```python
from build123d import *

# Parameters (mm, degrees)
SALIENTE_EXTRUIR1_DEPTH = 2
SALIENTE_EXTRUIR2_DEPTH = 24
CROQUIS4_W              = 26.838471133
CROQUIS4_H              = 17.040828642
CORTAR_EXTRUIR1_DEPTH   = 70.1
SALIENTE_EXTRUIR3_DEPTH = 2
SALIENTE_EXTRUIR4_DEPTH = 2
CROQUIS7_W              = 45.5
CROQUIS7_H              = 2
SALIENTE_EXTRUIR5_DEPTH = 8
SALIENTE_EXTRUIR6_DEPTH = 6
CROQUIS9_W              = 76.962380363
CROQUIS9_H              = 58.957858246
CORTAR_EXTRUIR2_DEPTH   = 39


with BuildPart() as part:
    # Croquis1 → Saliente-Extruir1 (new body)
    with BuildSketch(Plane.XY):
        Polygon((-48.939551095, 26.503456625), (-8.439551095, 26.503456625), (-4.439551095, 26.503456625), (-4.439551095, 1.503456625), (-8.439551095, 1.503456625), (-49.939551095, 1.503456625), (-49.939551095, 5.503456625), (-49.939551095, 26.503456625), align=None)
    extrude(amount=SALIENTE_EXTRUIR1_DEPTH)

    # Croquis3 → Saliente-Extruir2 (add)
    with BuildSketch(Plane.XY):
        Polygon((-48.939551095, 26.503456625), (-8.439551095, 26.503456625), (-4.439551095, 26.503456625), (-4.439551095, 1.503456625), (-49.939551095, 1.503456625), (-49.939551095, 26.503456625), align=None)
        Polygon((-10.439551095, 3.503456625), (-47.939551095, 3.503456625), (-47.939551095, 5.503456625), (-47.939551095, 24.503456625), (-10.439551095, 24.503456625), (-6.439551095, 24.503456625), (-6.439551095, 3.503456625), align=None, mode=Mode.SUBTRACT)
    extrude(amount=SALIENTE_EXTRUIR2_DEPTH)

    # Croquis4 → Cortar-Extruir1 (cut)
    with BuildSketch(Plane(origin=(0, 0, 0), x_dir=(0, 0, -1), z_dir=(1, 0, 0))):
        with Locations((-15.419235567, 13.92807924)):
            Rectangle(CROQUIS4_W, CROQUIS4_H)
    extrude(amount=-CORTAR_EXTRUIR1_DEPTH, mode=Mode.SUBTRACT)

    # Croquis5 → Saliente-Extruir3 (add)
    with BuildSketch(Plane(origin=(0, 26.503456625, 0), x_dir=(1, 0, 0), z_dir=(0, 1, 0))):
        Polygon((-49.939551095, -20.607192887), (-4.439551095, -20.607192887), (-4.439551095, -36.1), (-8.439551095, -36.1), (-48.939551095, -36.1), (-49.939551095, -36.1), align=None)
    extrude(amount=-SALIENTE_EXTRUIR3_DEPTH)

    # Croquis6 → Saliente-Extruir4 (add)
    with BuildSketch(Plane.XY.offset(36.1)):
        Polygon((-4.439551095, 24.503456625), (-49.939551095, 24.503456625), (-49.939551095, 33.503456625), (-49.939551095, 34.503456625), (-4.439551095, 34.503456625), (-4.439551095, 33.503456625), align=None)
    extrude(amount=-SALIENTE_EXTRUIR4_DEPTH)

    # Croquis7 → Saliente-Extruir5 (add)
    with BuildSketch(Plane.XY.offset(36.1)):
        with Locations((-27.189551095, 33.503456625)):
            Rectangle(CROQUIS7_W, CROQUIS7_H)
    extrude(amount=-SALIENTE_EXTRUIR5_DEPTH)

    # Croquis8 → Saliente-Extruir6 (add)
    with BuildSketch(Plane.XY.offset(36.1)):
        Polygon((-49.939551095, 29.503456625), (-49.939551095, 26.503456625), (-49.715027183, 26.503456625), (-8.439551095, 26.503456625), (-4.439551095, 26.503456625), (-4.439551095, 29.503456625), (-8.439551095, 29.503456625), (-49.715027183, 29.503456625), align=None)
    extrude(amount=-SALIENTE_EXTRUIR6_DEPTH)

    # Croquis9 → Cortar-Extruir2 (cut)
    with BuildSketch(Plane.XY.offset(24)):
        with Locations((-25.38769132, 23.863692023)):
            Rectangle(CROQUIS9_W, CROQUIS9_H)
    extrude(amount=-CORTAR_EXTRUIR2_DEPTH, mode=Mode.SUBTRACT)


solid = part.part
```
Here's how the part is built. I have some questions about the finished solid (model axes, mm). A direction names the side the tool comes from. Coordinates: 2 decimals unless noted, no trailing zeros. Order: outer loops, then holes, each group sorted by start corner. A loop starts at its lowest first (then second) coordinate and runs counter-clockwise, first axis right, second up. Notation, with made-up numbers: (85, 10) -> (89, 10) arc R18 cw to (89, 26) -> close; hole circle Ø2 at (54, 85). An arc over 180 degrees is marked (long way). Return JSON: item names as keys, results as strings.
1) On a 3-axis mill with a long thin cutter (end or side, diameter ignored), from which of +Z, -Z, +X, -X, +Y, -Y can I reach the whole of each face in a straight line? I mean faces 5 (the flat face through (-4.44, 28, 31)), 6 (the flat face through (-28, 34, 28.1)), 7 (the flat face through (-27, 29.503, 32)). Say none if no direction works.
Conclusion:
{"face 5": "+Z, -Z, +X, +Y, -Y", "face 6": "-Z, +X, -X, +Y", "face 7": "-Z, +X, -X"}
2) I'm going to push flat-ended pins straight in: P1, Ø2, axis at x = -27.5, y = 33.5, coming from the -Z side; P2, Ø1.5, axis at x = -11.5, y = 31, coming from the -Z side; P3, Ø1.5, axis at x = -29.5, y = 27.5, coming from the -Z side. Where does each tip first touch, or does it pass through?
Conclusion:
{"P1": "stops at z = 28.1", "P2": "stops at z = 34.1", "P3": "stops at z = 30.1"}
3) If I drill on probe 1 along Y at (x, z) = (-43, 33); probe 2 along Y at (x, z) = (-22.5, 28.25); probe 3 along Z at (x, y) = (-10.5, 31), over which ranges is the centre line in solid material (lowest first)?
Conclusion:
{"probe 1": "y = 24.5 to 29.5, 32.5 to 34.5", "probe 2": "y = 24.5 to 26.5, 32.5 to 34.5", "probe 3": "z = 34.1 to 36.1"}
4) If we section it at C-C on z = 33.25: List the corners of the cut face in (x, y) for me, plus the area to 4 significant figures.
Conclusion:
{"outline": "(-49.94, 24.5) -> (-4.44, 24.5) -> (-4.44, 29.5) -> (-49.94, 29.5) -> close; (-49.94, 32.5) -> (-4.44, 32.5) -> (-4.44, 34.5) -> (-49.94, 34.5) -> close", "area": "318.5 mm²"}
5) Thinking about a two-plate mould opening in Y: for faces 1 (the flat face through (-27, 26.503, 27)), 2 (the flat face through (-28, 30, 36.1)), 3 (the flat face through (-27, 24.503, 30)), 4 (the flat face through (-28, 34.503, 32)), which applies, +Y half, -Y half, draft (parallel to the pull), parting line (faces both ways), or undercut?
Conclusion:
{"face 1": "undercut", "face 2": "draft", "face 3": "-Y half", "face 4": "+Y half"}
6) If we section it at A-A on z = 28.5: List the corners of the cut face in (x, y) for me, plus the area to 3 significant figures.
Conclusion:
{"outline": "(-49.94, 24.5) -> (-4.44, 24.5) -> (-4.44, 26.5) -> (-49.94, 26.5) -> close; (-49.94, 32.5) -> (-4.44, 32.5) -> (-4.44, 34.5) -> (-49.94, 34.5) -> close", "area": "182 mm²"}
7) If we section it at B-B on x = -46.5: List the corners of the cut face in (y, z) for me, plus the area to 3 significant figures.
Conclusion:
{"outline": "(24.5, 24) -> (26.5, 24) -> (26.5, 30.1) -> (29.5, 30.1) -> (29.5, 34.1) -> (32.5, 34.1) -> (32.5, 28.1) -> (34.5, 28.1) -> (34.5, 36.1) -> (24.5, 36.1) -> close", "area": "64.2 mm²"}
8) If we section it at D-D on y = 30.5: List the corners of the cut face in (x, z) for me.
Conclusion:
{"outline": "(-49.94, 34.1) -> (-4.44, 34.1) -> (-4.44, 36.1) -> (-49.94, 36.1) -> close"}
